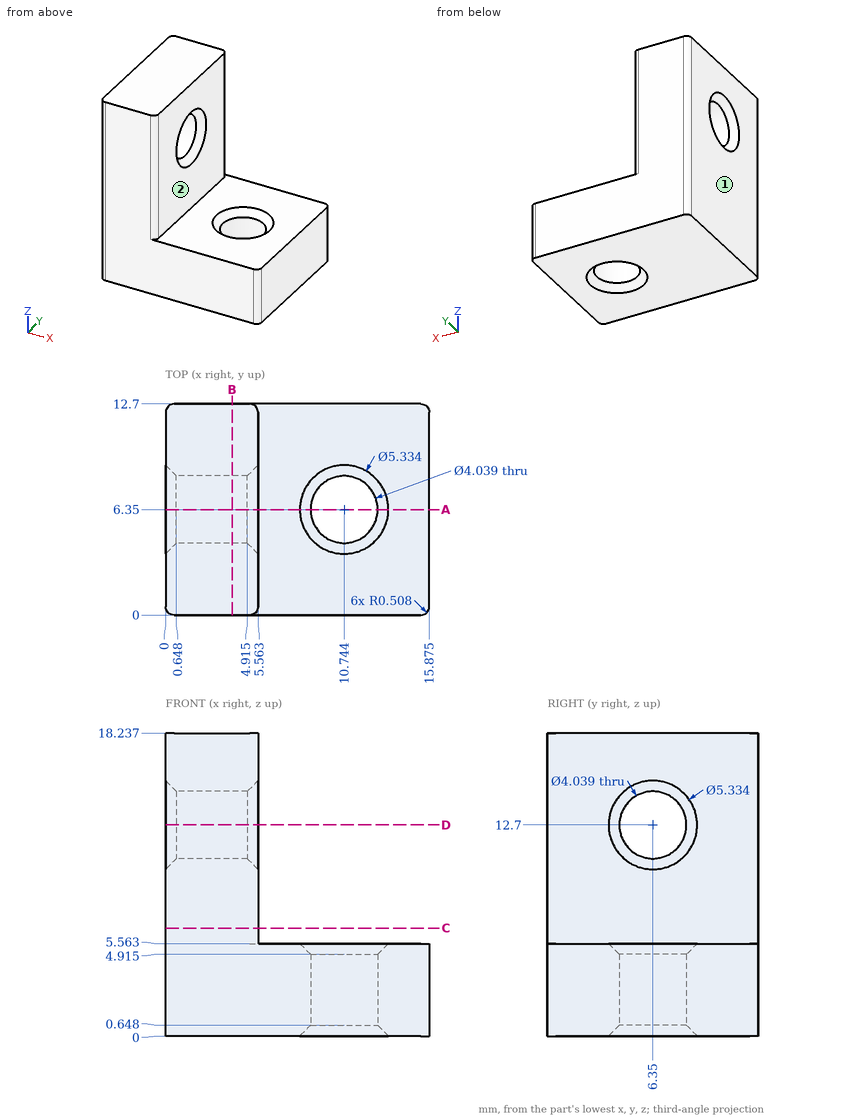
Design review of the part shown in the three views and the two pictorial views. Dimensions are in mm from the part's minimum x, y and z. A direction names the side the tool comes from. Coordinates: 2 decimals unless noted, no trailing zeros. Write each loop counter-clockwise with the first axis right and the second up, starting at its lowest first coordinate (ties: lowest second). Pieces come first, ordered by that corner, then holes.
1) We need section D-D on z = 12.7. State the section outline as (x, y) points (1 decimal), then the cut area to 3 significant figures.
2) To check wall thickness, follow probe 1 along Y at (x, z) = (2.9, 12.7); probe 2 along Z at (x, y) = (3.5, 6.35); probe 3 along Y at (x, z) = (2.25, 13.25). State the ranges of each line that lie inside material, in increasing order.
3) We need section C-C on z = 6.5. State the section outline as (x, y) points (1 decimal).
4) Machinability: for the marked faces 1 and 2, which of the approach directions +Z, -Z, +X, -X, +Y, -Y give a long, thin tool a straight path to every point of the face, cutting with its end or side? Answer none if there is none.
5) We need section A-A on y = 6.35. State the section outline as (x, z) points (1 decimal), then the cut area to 3 significant figures.
6) We need section B-B on x = 4. State the section outline as (y, z) points, then the cut area to 3 significant figures.
7) Clearance check with flat-ended pins moving along their axes: pin 1 Ø5.5 at (y, z) = (6.35, 12.7) entering from -X; pin 2 Ø6.5 at (x, y) = (10.74, 6.35) entering from +Z; pin 3 Ø3.5 at (y, z) = (4, 9.5) entering from +X. State where each tip first meets the part, or that it passes through.
Answer list:
1. outline: (0, 0.5) arc R0.5 ccw to (0.5, 0) - (5.1, 0) arc R0.5 ccw to (5.6, 0.5) - (5.6, 3.7) - (4.9, 4.3) - (0.6, 4.3) - (0, 3.7) - close; (0, 9) - (0.6, 8.4) - (4.9, 8.4) - (5.6, 9) - (5.6, 12.2) arc R0.5 ccw to (5.1, 12.7) - (0.5, 12.7) arc R0.5 ccw to (0, 12.2) - close
1. area: 47.1 mm2
2. probe 1: y = 0 to 4.33, 8.37 to 12.7
2. probe 2: z = 0 to 10.68, 14.72 to 18.24
2. probe 3: y = 0 to 4.41, 8.29 to 12.7
3. outline: (0, 0.5) arc R0.5 ccw to (0.5, 0) - (5.1, 0) arc R0.5 ccw to (5.6, 0.5) - (5.6, 12.2) arc R0.5 ccw to (5.1, 12.7) - (0.5, 12.7) arc R0.5 ccw to (0, 12.2) - close
4. face 1: +Z, -Z, -X, +Y, -Y
4. face 2: +Z, +X, +Y, -Y
5. outline: (0, 0) - (8.1, 0) - (8.7, 0.6) - (8.7, 4.9) - (8.1, 5.6) - (5.6, 5.6) - (5.6, 10) - (4.9, 10.7) - (0.6, 10.7) - (0, 10) - close; (0, 15.4) - (0.6, 14.7) - (4.9, 14.7) - (5.6, 15.4) - (5.6, 18.2) - (0, 18.2) - close; (12.8, 0.6) - (13.4, 0) - (15.9, 0) - (15.9, 5.6) - (13.4, 5.6) - (12.8, 4.9) - close
5. area: 112 mm2
6. outline: (0, 0) - (12.7, 0) - (12.7, 18.24) - (0, 18.24) - close; hole circle Ø4.04 at (6.35, 12.7)
6. area: 219 mm2
7. pin 1: stops at x = 0
7. pin 2: stops at z = 5.56
7. pin 3: stops at x = 5.56
